Input: part model. Units: mm. Frame: model coordinates. Face numbers are marked on the shaded views. Give positions to 0.01 mm unless a question says otherwise; leave off trailing zeros. Loops run counter-clockwise (first coordinate to the right, second up) from the corner with the lowest first, then second, coordinate; pieces in that order, holes last.
from build123d import *

# Parameters (mm, degrees)
SKETCH_R        = 50.5
PAD_DEPTH       = 5
SKETCH001_R     = 40.5
PAD001_DEPTH    = 5
SKETCH002_R     = 37
POCKET_DEPTH    = 5
POCKET001_DEPTH = 5
SKETCH004_R     = 2.05
POCKET002_DEPTH = 5
CHAMFER_SIZE    = 2
FILLET_R        = 1


with BuildPart() as part:
    # Sketch → Pad (new body)
    with BuildSketch(Plane.XY):
        Circle(SKETCH_R)
    extrude(amount=PAD_DEPTH)

    # Sketch001 (on Face3 of Pad) → Pad001 (join)
    with BuildSketch(Plane.XY.offset(5)):
        Circle(SKETCH001_R)
    extrude(amount=PAD001_DEPTH)

    # Sketch002 (on Face5 of Pad001) → Pocket (cut)
    with BuildSketch(Plane.XY.offset(10)):
        Circle(SKETCH002_R)
    extrude(amount=-POCKET_DEPTH, mode=Mode.SUBTRACT)

    # Sketch003 (on Face5 of Pocket) → Pocket001 (cut)
    with BuildSketch(Plane.XY.offset(10)):
        Polygon((26.870058, 31.112698), (31.112698, 26.870058), (26.870058, 22.627417), (22.627417, 26.870058), align=None)
    extrude(amount=-POCKET001_DEPTH, mode=Mode.SUBTRACT)

    # Sketch004 (on Face2 of Pocket001) → Pocket002 (cut)
    with BuildSketch(Plane(origin=(0, 0, 0), x_dir=(1, 0, 0), z_dir=(0, 0, -1))):
        with Locations((0, 45)):
            Circle(SKETCH004_R)
        with Locations((-45, 0)):
            Circle(SKETCH004_R)
        with Locations((45, 0)):
            Circle(SKETCH004_R)
        with Locations((0, -45)):
            Circle(SKETCH004_R)
    extrude(amount=-POCKET002_DEPTH, mode=Mode.SUBTRACT)

    # Chamfer
    chamfer_edges = [part.edges().sort_by_distance(p)[0] for p in [
        (42.95, 0, 0),
        (-2.05, 45, 0),
        (-47.05, 0, 0),
        (-2.05, -45, 0),
    ]]
    chamfer(chamfer_edges, length=CHAMFER_SIZE)

    # Fillet
    fillet_edges = [part.edges().sort_by_distance(p)[0] for p in [
        (-50.5, 0, 0),
        (-50.5, 0, 5),
    ]]
    fillet(fillet_edges, radius=FILLET_R)


solid = part.part
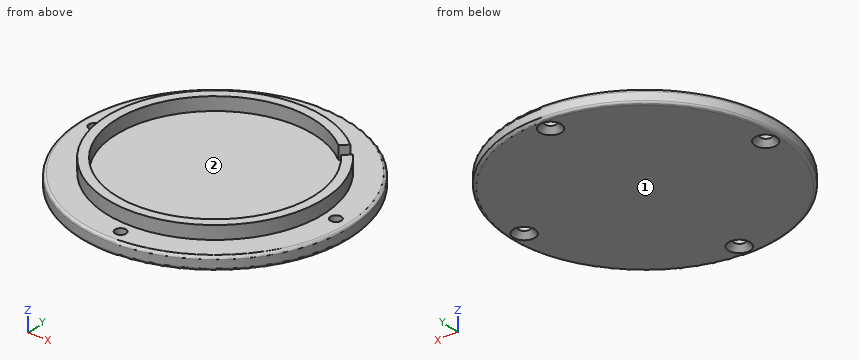
(1) Cut plane C-C (z = 8.25). Return the cut outline in (x, y), and give its area (3 significant figures).
Values follow:
outline: (23.96, 28.2) - (26.44, 30.68) arc R40.5 ccw (long way) to (30.68, 26.44) - (28.2, 23.96) arc R37 cw (long way) to start
area: 831 mm2
(2) Pin query (flat end, axial travel): pin 1 Ø2 at (y, z) = (4.5, 5.5) entering from -X; pin 2 Ø2 at (x, z) = (-22.5, 3.5) entering from +Y; pin 3 Ø1.5 at (x, y) = (12.5, -1) entering from +Z. Return the tip coordinate at first contact, or that it passes through.
Values follow:
pin 1: stops at x = -50.17
pin 2: stops at y = 45.69
pin 3: stops at z = 5
(3) Cut plane A-A (x = 0). Return the cut outline in (y, z), and give its area (3 significant figures).
Values follow:
outline: (-50.5, 1) arc R1 ccw to (-49.5, 0) - (-49.05, 0) - (-47.05, 2) - (-47.05, 5) - (-49.5, 5) arc R1 ccw to (-50.5, 4) - close; (-42.95, 2) - (-40.95, 0) - (40.95, 0) - (42.95, 2) - (42.95, 5) - (40.5, 5) - (40.5, 10) - (37, 10) - (37, 5) - (-37, 5) - (-37, 10) - (-40.5, 10) - (-40.5, 5) - (-42.95, 5) - close; (47.05, 2) - (49.05, 0) - (49.5, 0) arc R1 ccw to (50.5, 1) - (50.5, 4) arc R1 ccw to (49.5, 5) - (47.05, 5) - close
area: 490 mm2
(4) Mould query, pull axis X, two halves, no side actions, for the marked faces 1 and 2. Classes: +X half, -X half, draft (parallel to the pull), parting line (faces both ways), or undercut.
Values follow:
face 1: draft
face 2: undercut
(5) Ray query, probe 1 along Y at (x, z) = (0, 3.05); probe 2 along X at (y, z) = (0, 6.8); probe 3 along Z at (x, y) = (32.5, 10.5). Return the intervals inside material, ascending.
Values follow:
probe 1: y = -50.5 to -47.05, -42.95 to 42.95, 47.05 to 50.5
probe 2: x = -40.5 to -37, 37 to 40.5
probe 3: z = 0 to 5
